from build123d import *

# Parameters (mm, degrees)
SKETCH1_R           = 12.7
BOSS_EXTRUDE1_DEPTH = 304.8
SKETCH2_W           = 88.9
SKETCH2_H           = 38.1
BOSS_EXTRUDE2_DEPTH = 6.35


with BuildPart() as part:
    # Sketch1 → Boss-Extrude1 (new, symmetric)
    with BuildSketch(Plane(origin=(0, 0, 0), x_dir=(0, 0, -1), z_dir=(1, 0, 0))):
        with Locations(Location((0, 0, 0), (0, 0, 180))):
            Circle(SKETCH1_R)
    extrude(amount=BOSS_EXTRUDE1_DEPTH, both=True)

    # Sketch2 → Boss-Extrude2 (add)
    with BuildSketch(Plane(origin=(304.8, 0, 0), x_dir=(0, 0, -1), z_dir=(1, 0, 0))):
        with Locations((19.05, 0)):
            Rectangle(SKETCH2_W, SKETCH2_H)
    boss_extrude2 = extrude(amount=BOSS_EXTRUDE2_DEPTH)

    # Mirror1: Boss-Extrude2 across plane
    add(boss_extrude2.mirror(Plane(origin=(0, 0, 0), x_dir=(0, 0, 1), z_dir=(1, 0, 0))))


solid = part.part
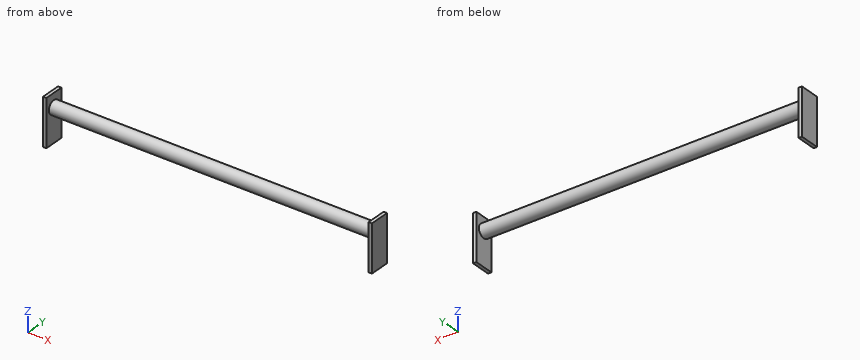
The listing builds one solid part. Answer for the finished solid, in the listing's coordinates (mm). Give positions to 0.01 mm unless a question says otherwise; leave off trailing zeros. Order: outer loops, then holes, each group sorted by start corner. A loop starts at its lowest first (then second) coordinate and runs counter-clockwise, first axis right, second up. Notation, with made-up numbers: (15.5, -17.75) - (25.5, -17.75) arc R13 ccw to (25.5, 2.25) - close; hole circle Ø9 at (76.25, -19). An arc over 180 degrees is marked (long way). One line per item, written item: value. Start each with the question number.
1) A cutting plane is placed at B-B on z = 0. Give the vertices of the cut face in (x, y), then the cut area to 3 significant figures.
2) Given pin 1 Ø6 at (x, z) = (-80.5, 0.5) entering from -Y; pin 2 Ø1.5 at (x, y) = (178, -12.5) entering from -Z; pin 3 Ø4 at (x, y) = (-174.5, -4) entering from -Z, each flat-ended and moving along its own axis, determine where each tip first touches the part or whether it passes through.
3) A cutting plane is placed at C-C on y = 0. Give the vertices of the cut face in (x, z), then the cut area to 3 significant figures.
4) Find the intervals of material crossed by L1, parallel to X at y = 10, z = -32.5; L2, parallel to Y at x = 135.5, z = -10.5; L3, parallel to Y at x = 236.5, z = 3, in increasing order.
5) A cutting plane is placed at A-A on z = -52.5. Give the vertices of the cut face in (x, y).
6) A cutting plane is placed at D-D on x = 82. Give the vertices of the cut face in (y, z).
Answer sheet:
1. outline: (-311.15, -19.05) - (-304.8, -19.05) - (-304.8, -12.7) - (304.8, -12.7) - (304.8, -19.05) - (311.15, -19.05) - (311.15, 19.05) - (304.8, 19.05) - (304.8, 12.7) - (-304.8, 12.7) - (-304.8, 19.05) - (-311.15, 19.05) - close
1. area: 16,000 mm2
2. pin 1: stops at y = -12.7
2. pin 2: stops at z = -4.82
2. pin 3: stops at z = -12.54
3. outline: (-311.15, -63.5) - (-304.8, -63.5) - (-304.8, -12.7) - (304.8, -12.7) - (304.8, -63.5) - (311.15, -63.5) - (311.15, 25.4) - (304.8, 25.4) - (304.8, 12.7) - (-304.8, 12.7) - (-304.8, 25.4) - (-311.15, 25.4) - close
3. area: 16,600 mm2
4. L1: x = -311.15 to -304.8, 304.8 to 311.15
4. L2: y = -7.14 to 7.14
4. L3: y = -12.34 to 12.34
5. outline: (-311.15, -19.05) - (-304.8, -19.05) - (-304.8, 19.05) - (-311.15, 19.05) - close; (304.8, -19.05) - (311.15, -19.05) - (311.15, 19.05) - (304.8, 19.05) - close
6. outline: circle Ø25.4 at (0, 0)
